from build123d import *

# Parameters (mm, degrees)
F2_R     = 9.525
F3_DEPTH = 11.6078
F5_D     = 6.35
F6_R     = 27.94


with BuildPart() as f1:
    # F0 (on Right) → F1 (revolve)
    with BuildSketch(Plane.YZ):
        Polygon((0, 15.875), (0, 0), (101.6, 0), (101.6, 15.875), (69.85, 15.875), (55.88, 11.7348), (48.26, 11.7348), (31.75, 15.875), align=None)
    revolve(axis=Axis((0, 35.272012, 0), (0, 1, 0)))

    # F2 (on face) → F3 (cut)
    with BuildSketch(Plane.XZ):
        Circle(F2_R)
    extrude(amount=-F3_DEPTH, mode=Mode.SUBTRACT)

    # F5 (through all)
    with Locations(Plane(origin=(0, 101.6, 0), x_dir=(-1, 0, 0), z_dir=(0, 1, 0))):
        with Locations((0, 0)):
            Hole(F5_D / 2)

    # F6
    f6_edges = [f1.edges().sort_by_distance(p)[0] for p in [
        (0, 48.26, -11.7348),
        (0, 55.88, -11.7348),
    ]]
    fillet(f6_edges, radius=F6_R)


solid = f1.part
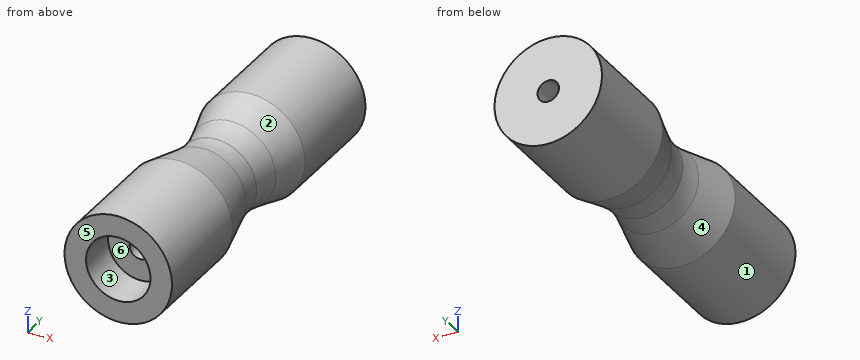
CAD build for the part. Positions are in the model's coordinates, mm. Face numbers are marked on the shaded views. A direction names the side the tool comes from. Round coordinates to 2 decimals unless told otherwise and drop trailing zeros. Order: outer loops, then holes, each group sorted by start corner. A loop starts at its lowest first (then second) coordinate and runs counter-clockwise, first axis right, second up. Notation, with made-up numbers: M 12,72.5 L 41,72.5 A26 ccw 41,99.5 Z; hole C 82.5,36 d2. An arc over 180 degrees is marked long. Use one line per item in the form item = value.
Q1. Saw through at B-B on y = 61.5. Give the cut face in (x, z) (3 decimals).
Recorded:
outline = C 0,0 d26.801; hole C 0,0 d6.35
Q2. Flat gauge pins, fed straight in: P1, Ø10, axis at y = 42.5, z = -1, coming from the +X side; P2, Ø10, axis at x = -7, y = 31.5, coming from the +Z side; P3, Ø10, axis at y = 30.5, z = 11.5, coming from the -X side; P4, Ø5, axis at x = 0, z = 0, coming from the +Y side. Where does each tip first touch, or does it go through?
Recorded:
P1 = 14.42
P2 = 15.75
P3 = -14.48
P4 = through
Q3. Two-plate mould, pull along Z, no slides. Class the marked faces 3, 4, 5 and 6: +Z half, -Z half, draft (parallel to the pull), parting line (faces both ways), or undercut.
Recorded:
face_3 = undercut
face_4 = parting line
face_5 = draft
face_6 = undercut
Q4. Probe L1, parallel to Y at x = -8, z = 0.5; L2, parallel to Z at x = 0, y = 46 (3 decimals); L3, parallel to Z at x = 0, y = 59 (3 decimals). List the from-to ranges inside material, lowest first.
Recorded:
L1 = 11.61 to 101.6
L2 = -12.324 to -3.175, 3.175 to 12.324
L3 = -12.671 to -3.175, 3.175 to 12.671
Q5. Saw through at A-A on y = 95.5. Give the cut face in (x, z) (3 decimals), then the cut area to 3 significant figures.
Recorded:
outline = C 0,0 d31.75; hole C 0,0 d6.35
area = 760 mm^2
Q6. Which spindle directions (+Z, -Z, +X, -X, +Y, -Y) get a long thin tool onto all of the face, cutting with end or side? Do the marked faces 1 and 2. Say none if no direction does.
Recorded:
face_1 = +Y, -Y
face_2 = none
